Build history of the part. All positions in model axes, mm. A direction names the side the tool comes from. Round coordinates to 2 decimals unless told otherwise and drop trailing zeros. Loops run counter-clockwise (first coordinate to the right, second up) from the corner with the lowest first, then second, coordinate; pieces in that order, holes last. Notation, with made-up numbers: M -37,66.25 L 1,66.25 A33 ccw 1,97.25 Z; hole C 30,-8.75 d3. An arc over 180 degrees is marked long. Use one line per item in the form item = value. Start each with the question number.
```python
from build123d import *

# Parameters (mm, degrees)
F0_W     = 220
F0_H     = 300
F1_DEPTH = 100
F2_W     = 215
F2_H     = 295
F3_DEPTH = 95
F4_W     = 215
F4_H     = 95
F5_DEPTH = 5
F6_SIZE  = 96


with BuildPart() as f1:
    # F0 (on Top) → F1 (new body)
    with BuildSketch(Plane.XY):
        Rectangle(F0_W, F0_H)
    extrude(amount=F1_DEPTH)

    # F2 (on face) → F3 (cut)
    with BuildSketch(Plane.XY.offset(100)):
        Rectangle(F2_W, F2_H)
    extrude(amount=-F3_DEPTH, mode=Mode.SUBTRACT)

    # F4 (on face) → F5 (cut)
    with BuildSketch(Plane.XZ.offset(-147.5)):
        with Locations((0, 52.5)):
            Rectangle(F4_W, F4_H)
    extrude(amount=-F5_DEPTH, mode=Mode.SUBTRACT)

    # F6
    f6_edges = [f1.edges().sort_by_distance(p)[0] for p in [
        (-108.75, 150, 100),
    ]]
    chamfer(f6_edges, length=F6_SIZE)


solid = f1.part
```
Q1. Tool access for faces 5 (the face through (-2, -147.5, 53)), 6 (the face through (110, -35, 49)): list every direction of +Z, -Z, +X, -X, +Y, -Y with a clear straight run to the whole face (end or side of a thin tool).
Q2. Pull direction X, two halves, no side cores. Call faces 1 (the face through (-2, -150, 49)), 2 (the face through (107.5, -34, 52)), 3 (the face through (-107.5, -34, 52)), 4 (the face through (-110, -35, 49)): pulls with the +X half, pulls with the -X half, needs draft (parallel to the pull), parting line crosses it, or undercut.
Q3. Saw through at B-B (z = 93.5). Give the cut face in (x, y).
Q4. Drop flat-ended pins along their axis: P1, Ø1, axis at x = 53, z = 59, coming from the +Y side; P2, Ø10, axis at x = -37, y = -44, coming from the +Z side. Give the stop position or say it passes through.
Q5. Wall check: probe 1 along X at (y, z) = (-111.5, 51); probe 2 along Z at (x, y) = (93, 0); probe 3 along Y at (x, z) = (30.5, 60.5). Give the ranges that are in metal, low to high.
Q6. Saw through at A-A (y = -35.5). Give the cut face in (x, z).
Q7. Saw through at C-C (x = -19). Give the cut face in (y, z).
Filled in:
q1.face_5 = +Z, +Y
q1.face_6 = +Z, -Z, +X, +Y, -Y
q2.face_1 = needs draft
q2.face_2 = undercut
q2.face_3 = undercut
q2.face_4 = pulls with the -X half
q3.outline = M -110,-150 L 110,-150 L 110,60.5 L 107.5,60.5 L 107.5,-147.5 L -107.5,-147.5 L -107.5,60.5 L -110,60.5 Z
q4.P1 = -147.5
q4.P2 = 5
q5.probe_1 = -110 to -107.5, 107.5 to 110
q5.probe_2 = 0 to 5
q5.probe_3 = -150 to -147.5
q6.outline = M -110,0 L 110,0 L 110,100 L 107.5,100 L 107.5,5 L -107.5,5 L -107.5,100 L -110,100 Z
q7.outline = M -150,0 L 150,0 L 150,4 L 149,5 L -147.5,5 L -147.5,100 L -150,100 Z
